```python
from build123d import *

# Parameters (mm, degrees)
SKETCH1_W           = 99
SKETCH1_H           = 50.8
BOSS_EXTRUDE1_DEPTH = 5
SKETCH3_W           = 59
SKETCH3_H           = 41.5
BOSS_EXTRUDE2_DEPTH = 5
SKETCH2_R           = 3.175
CUT_EXTRUDE1_DEPTH  = 56.860630143
SKETCH4_R           = 2
BOSS_EXTRUDE3_DEPTH = 2.5
SKETCH5_R           = 1.25
CUT_EXTRUDE2_DEPTH  = 12
SKETCH6_W           = 6
SKETCH6_H           = 2
CUT_EXTRUDE3_DEPTH  = 2
SKETCH7_W           = 2
SKETCH7_H           = 6
CUT_EXTRUDE4_DEPTH  = 2


with BuildPart() as part:
    # Sketch1 → Boss-Extrude1 (new body)
    with BuildSketch(Plane.XY):
        Rectangle(SKETCH1_W, SKETCH1_H)
    extrude(amount=BOSS_EXTRUDE1_DEPTH)

    # Sketch3 → Boss-Extrude2 (add)
    with BuildSketch(Plane.XY.offset(5)):
        Rectangle(SKETCH3_W, SKETCH3_H)
    extrude(amount=BOSS_EXTRUDE2_DEPTH)

    # Sketch2 → Cut-Extrude1 (cut, through all)
    with BuildSketch(Plane.XY.offset(5)):
        with Locations((-39.5, 12.7)):
            Circle(SKETCH2_R)
        with Locations((-39.5, -12.7)):
            Circle(SKETCH2_R)
        with Locations((39.5, -12.7)):
            Circle(SKETCH2_R)
        with Locations((39.5, 12.7)):
            Circle(SKETCH2_R)
    extrude(amount=-CUT_EXTRUDE1_DEPTH, mode=Mode.SUBTRACT)

    # Sketch4 → Boss-Extrude3 (add)
    with BuildSketch(Plane.XY.offset(10)):
        with Locations(Location((-10.5, -18.25, 0), (0, 0, 180))):
            Circle(SKETCH4_R)
        with Locations(Location((9.5, -18.25, 0), (0, 0, 180))):
            Circle(SKETCH4_R)
        with Locations(Location((-10.5, 18.25, 0), (0, 0, 180))):
            Circle(SKETCH4_R)
        with Locations(Location((27, 18.25, 0), (0, 0, 180))):
            Circle(SKETCH4_R)
    extrude(amount=BOSS_EXTRUDE3_DEPTH)

    # Sketch5 → Cut-Extrude2 (cut)
    with BuildSketch(Plane.XY.offset(12.5)):
        with Locations((-10.5, 18.25)):
            Circle(SKETCH5_R)
        with Locations((27, 18.25)):
            Circle(SKETCH5_R)
        with Locations((9.5, -18.25)):
            Circle(SKETCH5_R)
        with Locations((-10.5, -18.25)):
            Circle(SKETCH5_R)
    extrude(amount=-CUT_EXTRUDE2_DEPTH, mode=Mode.SUBTRACT)

    # Sketch6 → Cut-Extrude3 (cut)
    with BuildSketch(Plane(origin=(0, -25.4, 0), x_dir=(-1, 0, 0), z_dir=(0, -1, 0))):
        with Locations((0, -4)):
            Rectangle(SKETCH6_W, SKETCH6_H)
    cut_extrude3 = extrude(amount=-CUT_EXTRUDE3_DEPTH, mode=Mode.SUBTRACT)

    # Sketch7 → Cut-Extrude4 (cut)
    with BuildSketch(Plane.ZY.offset(49.5)):
        with Locations((4, 0)):
            Rectangle(SKETCH7_W, SKETCH7_H)
    cut_extrude4 = extrude(amount=-CUT_EXTRUDE4_DEPTH, mode=Mode.SUBTRACT)

    # Mirror1: Cut-Extrude3 across plane
    add(cut_extrude3.mirror(Plane.ZX), mode=Mode.SUBTRACT)

    # Mirror2: Cut-Extrude4 across plane
    add(cut_extrude4.mirror(Plane(origin=(0, 0, 0), x_dir=(0, 0, 1), z_dir=(1, 0, 0))), mode=Mode.SUBTRACT)


solid = part.part
```
Could you check a few things on this model? Use its own coordinates, in mm. A direction names the side the tool comes from. Give positions to 0.01 mm unless a question says otherwise; leave off trailing zeros. Order: outer loops, then holes, each group sorted by start corner. A loop starts at its lowest first (then second) coordinate and runs counter-clockwise, first axis right, second up.
Q1. For faces 5 (the cylindrical face through (8.25, -18.2, 6.58)), 6 (the flat face through (0, 23.4, 4)), 7 (the flat face through (-29.5, 0, 7)), 8 (the flat face through (0, 20.75, 7)), 9 (the flat face through (-49, 3, 4)), which set-ups out of +Z, -Z, +X, -X, +Y, -Y let a thin tool reach every point of the face, with its end or its side?
Q2. Suppose I cut it at D-D, the plane z = 2. Count the separate pieces of the cut face and the enclosed holes in it, and give its area (3 significant figures).
Q3. I'm going to push flat-ended pins straight in: P1, Ø6, axis at x = -36, y = 7, coming from the +Z side; P2, Ø0.6, axis at x = 0, z = 3.5, coming from the -Y side; P3, Ø2, axis at x = -10.5, y = 18.25, coming from the +Z side. Where does each tip first touch, or does it pass through?
Q4. We'd pull the mould along X, two halves only. Please class faces 1 (the cylindrical face through (42.43, 11.48, 2.54)), 2 (the flat face through (8, -18, 12.5)), 3 (the flat face through (47.5, 0, 4)), 4 (the cylindrical face through (-10.24, 16.267, 11.232)): +X half, -X half, draft (parallel to the pull), parting line (faces both ways), or undercut.
Q5. Suppose I cut it at C-C, the plane x = -39. Write out the boundary of the cut face in (y, z).
Q6. Suppose I cut it at A-A, the plane z = 11.5. Write out the boundary of the cut face in (x, y).
Q7. Suppose I cut it at B-B, the plane y = -12.7. Write out the boundary of the cut face in (x, z) (3 decimals).
Q8. If I drill on line 1 along Y through (x, z) = (39.5, 2.4) (3 decimals); line 2 along X through (y, z) = (10.5, 2.5); line 3 along X through (y, z) = (5, 5.5), over which ranges is the centre line in solid material (lowest first)?
Solution:
1. face 5: +Z
1. face 6: +Z, +Y
1. face 7: +Z, -X, +Y, -Y
1. face 8: +Z, +X, -X, +Y
1. face 9: +Z, -X
2. separate pieces: 1
2. enclosed holes: 8
2. area: 4,880 mm2
3. P1: stops at z = 5
3. P2: stops at y = -23.4
3. P3: stops at z = 0.5
4. face 1: undercut
4. face 2: draft
4. face 3: +X half
4. face 4: undercut
5. outline: (-25.4, 0) - (-15.84, 0) - (-15.84, 5) - (-25.4, 5) - close; (-9.56, 0) - (9.56, 0) - (9.56, 5) - (-9.56, 5) - close; (15.84, 0) - (25.4, 0) - (25.4, 5) - (15.84, 5) - close
6. outline: circle Ø4 at (-10.5, -18.25); circle Ø4 at (-10.5, 18.25); circle Ø4 at (9.5, -18.25); circle Ø4 at (27, 18.25); hole circle Ø2.5 at (-10.5, -18.25); hole circle Ø2.5 at (-10.5, 18.25); hole circle Ø2.5 at (9.5, -18.25); hole circle Ø2.5 at (27, 18.25)
7. outline: (-49.5, 0) - (-42.675, 0) - (-42.675, 5) - (-49.5, 5) - close; (-36.325, 0) - (36.325, 0) - (36.325, 5) - (29.5, 5) - (29.5, 10) - (-29.5, 10) - (-29.5, 5) - (-36.325, 5) - close; (42.675, 0) - (49.5, 0) - (49.5, 5) - (42.675, 5) - close
8. line 1: y = -25.4 to -15.875, -9.525 to 9.525, 15.875 to 25.4
8. line 2: x = -49.5 to -41.79, -37.21 to 37.21, 41.79 to 49.5
8. line 3: x = -29.5 to 29.5
